For this review, take the finished solid that the model builds, in its own axes (mm). Face numbers are marked on the shaded views. A direction names the side the tool comes from. Round coordinates to 2 decimals unless told otherwise and drop trailing zeros. Write each loop counter-clockwise with the first axis right and the second up, starting at its lowest first coordinate (ties: lowest second). Pieces come first, ordered by that corner, then holes. Notation, with made-up numbers: M 75.25,58 L 132.25,58 A13 cw 132.25,82 Z; hole C 29,0.25 d3. An arc over 180 degrees is marked long. Write each question's results on one line, items separated by ' | '. Start each with the question number.
```python
from build123d import *

# Parameters (mm, degrees)
CUT_EXTRUDE1_DEPTH                               = 27.438608133
SKETCH3_W                                        = 19
SKETCH3_H                                        = 6.025
CBORE_FOR_M2_HEX_HEAD_MACHINE_SCREW2_D           = 2.459
CBORE_FOR_M2_HEX_HEAD_MACHINE_SCREW2_DEPTH       = 27.463932023
CBORE_FOR_M2_HEX_HEAD_MACHINE_SCREW2_CBORE_D     = 4
CBORE_FOR_M2_HEX_HEAD_MACHINE_SCREW2_CBORE_DEPTH = 23.263932023
FILLET1_R                                        = 0.2


with BuildPart() as part:
    # Sketch1 → Revolve1 (revolve)
    with BuildSketch(Plane(origin=(0, 0, 0), x_dir=(-1, 0, 0), z_dir=(0, 0, -1)), mode=Mode.PRIVATE) as revolve1_sk:
        Polygon((-9.5, 10), (-9.5, 0), (9.5, 0), (9.5, 10), (7.5, 10), (7.5, 13), (-7.5, 13), (-7.5, 10), align=None)
    revolve(revolve1_sk.sketch.rotate(Axis((9.5, 0, 0), (-1, 0, 0)), 270), axis=Axis((9.5, 0, 0), (-1, 0, 0)))

    # Sketch2 → Cut-Extrude1 (cut, through all)
    with BuildSketch(Plane.ZY.offset(9.5)):
        with BuildLine():
            Line((2.05, 5.638927203), (2.05, 7.8))
            Line((2.05, 7.8), (-2.05, 7.8))
            Line((-2.05, 7.8), (-2.05, 5.638927203))
            ThreePointArc((-2.05, 5.638927203), (0, 6), (2.05, 5.638927203))
        make_face()
    extrude(amount=-CUT_EXTRUDE1_DEPTH, mode=Mode.SUBTRACT)

    # Sketch3 → 0.5mm clearance (revolve, cut)
    with BuildSketch(Plane(origin=(0, 0, 0), x_dir=(-1, 0, 0), z_dir=(0, 0, -1))):
        with Locations((0, 3.0125)):
            Rectangle(SKETCH3_W, SKETCH3_H)
    revolve(axis=Axis((9.5, 0, 0), (-1, 0, 0)), mode=Mode.SUBTRACT)

    # CBORE for M2 Hex Head Machine Screw2
    with Locations(Plane(origin=(0, 35.263932023, 0), x_dir=(1, 0, 0), z_dir=(0, 1, 0))):
        with Locations((0, 0)):
            CounterBoreHole(CBORE_FOR_M2_HEX_HEAD_MACHINE_SCREW2_D / 2, CBORE_FOR_M2_HEX_HEAD_MACHINE_SCREW2_CBORE_D / 2, CBORE_FOR_M2_HEX_HEAD_MACHINE_SCREW2_CBORE_DEPTH, depth=CBORE_FOR_M2_HEX_HEAD_MACHINE_SCREW2_DEPTH)

    # Fillet1
    fillet1_edges = [part.edges().sort_by_distance(p)[0] for p in [
        (0, 7.8, -2.05),
        (0, 7.8, 2.05),
    ]]
    fillet(fillet1_edges, radius=FILLET1_R)


solid = part.part
```
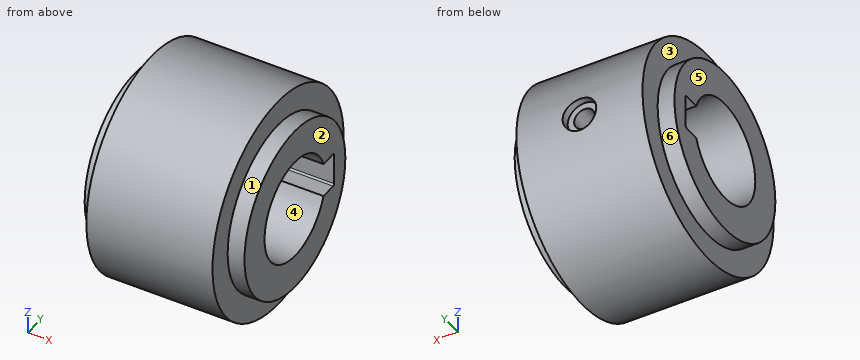
Item 1: We need section B-B on y = 0. State the section outline as (x, z) points (3 decimals), then the cut area to 3 significant figures.
Item 2: Insertion check: P1, Ø0.6, axis at x = -1.5, y = 6, coming from the -Z side; P2, Ø7, axis at y = 0, z = 0, coming from the -X side; P3, Ø1.5, axis at x = 1, y = -3.5, coming from the -Z side; P4, Ø3, axis at x = 0.5, z = -8, coming from the +Y side. Each pin has a flat end and moves straight along its axis. Give the tip position at first contact, or say it passes through.
Item 3: We need section D-D on z = -3.5. State the section outline as (x, y) points, then the cut area to 3 significant figures.
Item 4: Mouldability with a two-part tool opening along Z and no side actions: class the marked faces 4, 5 and 6 as pulls with the +Z half, pulls with the -Z half, needs draft (parallel to the pull), parting line crosses it, or undercut.
Item 5: For the marked faces 1, 2 and 3, list the 3-axis set-ups (+Z, -Z, +X, -X, +Y, -Y) from which the entire face can be reached by the end or side of a thin tool; tool diameter is ignored.
Item 6: We need section C-C on z = 0. State the section outline as (x, y) points (1 decimal), then the cut area to 3 significant figures.
Item 7: We need section A-A on x = 6.25. State the section outline as (y, z) points (3 decimals).
Item 8: For probe 1 along X at (y, z) = (5.75, -11.5); probe 2 along Z at (x, y) = (3.5, 2.75); probe 3 along Z at (x, y) = (-6, 4.5), list the stretches that pass through material, from the lowest coordinate up.
Numbers:
1) outline: M -9.5,-10 L -7.5,-10 L -7.5,-13 L 7.5,-13 L 7.5,-10 L 9.5,-10 L 9.5,-6.025 L -9.5,-6.025 Z; M -9.5,6.025 L 9.5,6.025 L 9.5,10 L 7.5,10 L 7.5,13 L -7.5,13 L -7.5,10 L -9.5,10 Z | area: 241 mm^2
2) P1: stops at z = -11.68 | P2: passes through | P3: stops at z = -12.71 | P4: stops at y = 11.26
3) outline: M -9.5,-9.37 L -7.5,-9.37 L -7.5,-12.52 L 7.5,-12.52 L 7.5,-9.37 L 9.5,-9.37 L 9.5,-4.9 L -9.5,-4.9 Z; M -9.5,4.9 L 9.5,4.9 L 9.5,9.37 L 7.5,9.37 L 7.5,12.52 L -7.5,12.52 L -7.5,9.37 L -9.5,9.37 Z | area: 264 mm^2
4) face 4: undercut | face 5: needs draft | face 6: parting line crosses it
5) face 1: +X | face 2: +Z, -Z, +X, +Y, -Y | face 3: -X
6) outline: M -9.5,-10 L -7.5,-10 L -7.5,-13 L 7.5,-13 L 7.5,-10 L 9.5,-10 L 9.5,-6 L -9.5,-6 Z; M -9.5,7.8 L -1.2,7.8 L -1.2,12 L -2,12 L -2,13 L -7.5,13 L -7.5,10 L -9.5,10 Z; M 1.2,7.8 L 9.5,7.8 L 9.5,10 L 7.5,10 L 7.5,13 L 2,13 L 2,12 L 1.2,12 Z | area: 193 mm^2
7) outline: C 0,0 d26; hole M 5.666,-2.05 L 7.6,-2.05 A0.2 ccw 7.8,-1.85 L 7.8,1.85 A0.2 ccw 7.6,2.05 L 5.666,2.05 A6.025 ccw long Z
8) probe 1: x = -7.5 to 7.5 | probe 2: z = -12.71 to -5.36, 5.36 to 12.71 | probe 3: z = -12.2 to -4.01, 4.01 to 12.2
